For this review, take the finished solid that the model builds, in its own axes (mm). A direction names the side the tool comes from. Coordinates: 2 decimals unless noted, no trailing zeros. Loops run counter-clockwise (first coordinate to the right, second up) from the corner with the lowest first, then second, coordinate; pieces in that order, holes last. Notation, with made-up numbers: M 11.5,-25.75 L 18.5,-25.75 A19 ccw 18.5,5.25 Z; hole C 64,-5.5 d5. An arc over 180 degrees is marked long. Put each result on its own line as item: value.
```python
from build123d import *

# Parameters (mm, degrees)
SKETCH1_W               = 320
SKETCH1_H               = 200
SKETCH1_W_2             = 280
SKETCH1_H_2             = 160
BOSS_EXTRUDE1_DEPTH     = 20
SKETCH2_W               = 130
SKETCH2_H               = 200
CUT_EXTRUDE1_DEPTH      = 20
SKETCH5_W               = 20
SKETCH5_H               = 20
BOSS_EXTRUDE4_DEPTH     = 40
SKETCH8_W               = 10
SKETCH8_H               = 14
BOSS_EXTRUDE5_DEPTH     = 20
SKETCH9_W               = 10
SKETCH9_H               = 14
BOSS_EXTRUDE6_DEPTH     = 20
SKETCH10_W              = 10
SKETCH10_H              = 10
BOSS_EXTRUDE7_DEPTH     = 20
SKETCH11_R              = 3
CUT_EXTRUDE2_DEPTH      = 30
SKETCH13_R              = 3
CUT_EXTRUDE3_DEPTH      = 30
CUT_EXTRUDE4_DEPTH      = 297.141857899
CUT_EXTRUDE4_DEPTH_BACK = 297.141857899
SKETCH14_R              = 3
CUT_EXTRUDE5_DEPTH      = 293.788319439
CUT_EXTRUDE5_DEPTH_BACK = 293.788319439
SKETCH16_R              = 3
SKETCH17_W              = 14
SKETCH17_H              = 38
CUT_EXTRUDE6_DEPTH      = 5
CUT_EXTRUDE7_DEPTH      = 1


with BuildPart() as part:
    # Sketch1 → Boss-Extrude1 (new body)
    with BuildSketch(Plane(origin=(0, 0, 0), x_dir=(1, 0, 0), z_dir=(0, 1, 0))):
        with Locations((160, 100)):
            Rectangle(SKETCH1_W, SKETCH1_H)
        with Locations((160, 100)):
            Rectangle(SKETCH1_W_2, SKETCH1_H_2, mode=Mode.SUBTRACT)
    extrude(amount=BOSS_EXTRUDE1_DEPTH)

    # Sketch2 → Cut-Extrude1 (cut)
    with BuildSketch(Plane(origin=(0, 20, 0), x_dir=(1, 0, 0), z_dir=(0, 1, 0))):
        with Locations((255, 100)):
            Rectangle(SKETCH2_W, SKETCH2_H)
    extrude(amount=-CUT_EXTRUDE1_DEPTH, mode=Mode.SUBTRACT)

    # Sketch5 → Boss-Extrude4 (add)
    with BuildSketch(Plane.XZ):
        with Locations((10, -10)):
            Rectangle(SKETCH5_W, SKETCH5_H)
        with Locations((10, -190)):
            Rectangle(SKETCH5_W, SKETCH5_H)
    extrude(amount=BOSS_EXTRUDE4_DEPTH)

    # Sketch8 → Boss-Extrude5 (add)
    with BuildSketch(Plane.XZ.offset(40)):
        with Locations((10, -10)):
            Rectangle(SKETCH8_W, SKETCH8_H)
    extrude(amount=BOSS_EXTRUDE5_DEPTH)

    # Sketch9 → Boss-Extrude6 (add)
    with BuildSketch(Plane.XZ.offset(40)):
        with Locations((10, -190)):
            Rectangle(SKETCH9_W, SKETCH9_H)
    extrude(amount=BOSS_EXTRUDE6_DEPTH)

    # Sketch10 → Boss-Extrude7 (add)
    with BuildSketch(Plane(origin=(190, 0, 0), x_dir=(0, 0, -1), z_dir=(1, 0, 0))):
        with Locations((190, 10)):
            Rectangle(SKETCH10_W, SKETCH10_H)
        with Locations((10, 10)):
            Rectangle(SKETCH10_W, SKETCH10_H)
    extrude(amount=BOSS_EXTRUDE7_DEPTH)

    # Sketch11 → Cut-Extrude2 (cut)
    with BuildSketch(Plane(origin=(0, 20, 0), x_dir=(1, 0, 0), z_dir=(0, 1, 0))):
        with Locations(Location((142.5, 190, 0), (0, 0, 270))):
            Circle(SKETCH11_R)
        with Locations(Location((95, 190, 0), (0, 0, 270))):
            Circle(SKETCH11_R)
        with Locations(Location((10, 100, 0), (0, 0, 270))):
            Circle(SKETCH11_R)
        with Locations(Location((142.5, 10, 0), (0, 0, 90))):
            Circle(SKETCH11_R)
        with Locations(Location((95, 10, 0), (0, 0, 90))):
            Circle(SKETCH11_R)
    extrude(amount=-CUT_EXTRUDE2_DEPTH, mode=Mode.SUBTRACT)

    # Sketch13 → Cut-Extrude3 (cut)
    with BuildSketch(Plane.ZY):
        with Locations((-8.2, -50)):
            Circle(SKETCH13_R)
        with Locations((-67, 11.8)):
            Circle(SKETCH13_R)
        with Locations((-133, 11.8)):
            Circle(SKETCH13_R)
        with Locations((-191.8, -50)):
            Circle(SKETCH13_R)
    extrude(amount=-CUT_EXTRUDE3_DEPTH, mode=Mode.SUBTRACT)

    # Sketch14 → Cut-Extrude4 (cut, two sides: drawn at the far end of the back side and taken through both)
    with BuildSketch(Plane(origin=(0, 0, -200), x_dir=(-1, 0, 0), z_dir=(0, 0, -1)).offset(-CUT_EXTRUDE4_DEPTH_BACK)):
        with Locations((-160, 10)):
            Circle(SKETCH14_R)
        with Locations((-30, 10)):
            Circle(SKETCH14_R)
        with Locations((-130, 10)):
            Circle(SKETCH14_R)
        with Locations((-70, 10)):
            Circle(SKETCH14_R)
    extrude(amount=CUT_EXTRUDE4_DEPTH + CUT_EXTRUDE4_DEPTH_BACK, mode=Mode.SUBTRACT)

    # Sketch16 → Cut-Extrude5 (cut, two sides: drawn at the far end of the back side and taken through both)
    with BuildSketch(Plane.XY.offset(-5).offset(-CUT_EXTRUDE5_DEPTH_BACK)):
        with Locations((200, 10)):
            Circle(SKETCH16_R)
    extrude(amount=CUT_EXTRUDE5_DEPTH + CUT_EXTRUDE5_DEPTH_BACK, mode=Mode.SUBTRACT)

    # Sketch17 → Cut-Extrude6 (cut)
    with BuildSketch(Plane(origin=(20, 0, 0), x_dir=(0, 0, -1), z_dir=(1, 0, 0))):
        with Locations((7, -21)):
            Rectangle(SKETCH17_W, SKETCH17_H)
    extrude(amount=-CUT_EXTRUDE6_DEPTH, mode=Mode.SUBTRACT)

    # Sketch18 → Cut-Extrude7 (cut)
    with BuildSketch(Plane(origin=(15, 0, 0), x_dir=(0, 0, -1), z_dir=(1, 0, 0))):
        Polygon((0, -2), (14, -2), (14, -40), (17, -40), (17, -60), (3, -60), (3, -40), (0, -40), align=None)
    extrude(amount=-CUT_EXTRUDE7_DEPTH, mode=Mode.SUBTRACT)


solid = part.part
```
(1) Wall thickness on line 1 along Z through (x, y) = (142.5, 14); line 2 along X through (y, z) = (10, -186); line 3 along Z through (x, y) = (87, 4): over which ranges is each line inside the solid? List them lowest first. Write a range as [from, to].
Determined:
line 1: z = [-200, -193], [-187, -180], [-20, -13], [-7, 0]
line 2: x = [0, 27], [33, 67], [73, 127], [133, 157], [163, 197], [203, 210]
line 3: z = [-200, -180], [-20, 0]
(2) Tool access review of faces 1 (the flat face through (200, 5, -10)), 2 (the flat face through (210, 10, -10)), 3 (the flat face through (200, 15, -10)): name each direction out of +Z, -Z, +X, -X, +Y, -Y from which nothing blocks a thin tool from reaching the whole face with its end or side.
Determined:
face 1: +Z, -Z, +X, -Y
face 2: +Z, -Z, +X, +Y, -Y
face 3: +Z, -Z, +X, +Y
(3) Add section B-B (y = -25.5). Write out the cut boundary in (x, z), plus the area to 3 significant figures.
Determined:
outline: M 0,-200 L 20,-200 L 20,-180 L 0,-180 Z; M 0,-20 L 20,-20 L 20,-14 L 14,-14 L 14,0 L 0,0 Z
area: 716 mm^2
(4) Draft analysis for pull direction Z (two halves, no side actions). For faces 4 (the flat face through (197.6, 7.7, -195)), 5 (the flat face through (14, 0, -101)), 6 (the flat face through (200, 15, -190)), 7 (the flat face through (9, -50, -3)), state which applies: +Z half, -Z half, draft (parallel to the pull), parting line (faces both ways), or undercut.
Determined:
face 4: -Z half
face 5: undercut
face 6: draft
face 7: +Z half
(5) Add section D-D (z = -67). Write out the cut boundary in (x, y), plus the area to 3 significant figures.
Determined:
outline: M 0,0 L 20,0 L 20,8.8 L 0,8.8 Z; M 0,14.8 L 20,14.8 L 20,20 L 0,20 Z
area: 280 mm^2
(6) Add section A-A (x = 10). Write out the cut boundary in (y, z).
Determined:
outline: M -60,-197 L -40,-197 L -40,-200 L 20,-200 L 20,-103 L 0,-103 L 0,-180 L -40,-180 L -40,-183 L -60,-183 Z; M -60,-17 L -40,-17 L -40,-20 L 0,-20 L 0,-97 L 20,-97 L 20,0 L -40,0 L -40,-3 L -60,-3 Z; hole C -50,-191.8 d6; hole C -50,-8.2 d6; hole C 11.8,-133 d6; hole C 11.8,-67 d6
(7) For pin 1 (8 mm diameter, centred on x = 11, y = -47, fed in from -Z); pin 2 (2 mm diameter, centred on y = 7.5, z = -121, fed in from +X); pin 3 (3.5 mm diameter, centred on x = 95, z = -190, fed in from -Y); pin 4 (1.8 mm diameter, centred on x = 17, z = -10.5, fed in from -Y), all flat-tipped, find the tip position at first contact; note any pin that passes through.
Determined:
pin 1: stops at z = -197
pin 2: stops at x = 20
pin 3: passes through
pin 4: stops at y = -2
(8) Add section C-C (x = 77). Write out the cut boundary in (y, z), plus the area to 3 significant figures.
Determined:
outline: M 0,-200 L 20,-200 L 20,-180 L 0,-180 Z; M 0,-20 L 20,-20 L 20,0 L 0,0 Z
area: 800 mm^2
